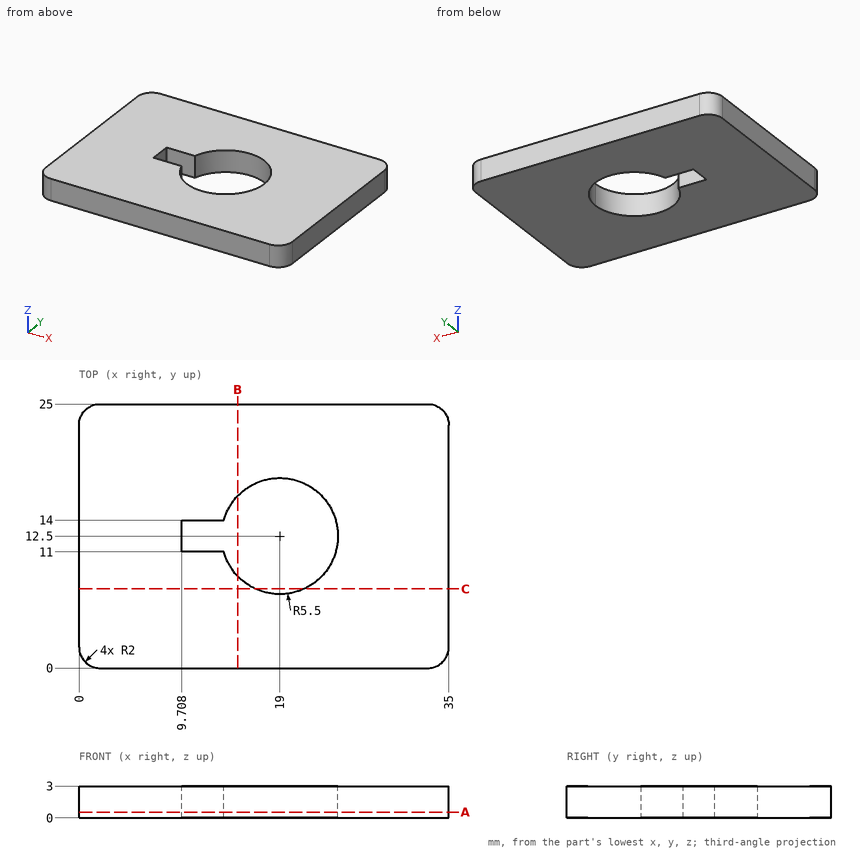
Could you check a few things on this drawing? It's one solid part, dimensions in mm from its lowest x, y, z. Give positions to 0.01 mm unless a question says otherwise; leave off trailing zeros. Write each loop counter-clockwise with the first axis right and the second up, starting at its lowest first coordinate (ties: lowest second). Pieces come first, ordered by that corner, then holes.
(1) If I drill on L1, parallel to X at y = 12.25, z = 2.3 (1 decimal); L2, parallel to Y at x = 19, z = 2.35; L3, parallel to X at y = 13.25, z = 2.05, over which ranges is the centre line in solid material (lowest first)?
Output values:
L1: x = 0 to 9.7, 24.5 to 35
L2: y = 0 to 7, 18 to 25
L3: x = 0 to 9.71, 24.45 to 35
(2) Imagine slicing it at C-C, the plane y = 7.5. Write out the boundary of the cut face in (x, z).
Output values:
outline: (0, 0) - (16.71, 0) - (16.71, 3) - (0, 3) - close; (21.29, 0) - (35, 0) - (35, 3) - (21.29, 3) - close
(3) Imagine slicing it at B-B, the plane x = 15. Write out the boundary of the cut face in (y, z) (1 decimal).
Output values:
outline: (0, 0) - (8.7, 0) - (8.7, 3) - (0, 3) - close; (16.3, 0) - (25, 0) - (25, 3) - (16.3, 3) - close
(4) Imagine slicing it at A-A, the plane z = 0.55. Write out the boundary of the cut face in (x, y).
Output values:
outline: (0, 2) arc R2 ccw to (2, 0) - (33, 0) arc R2 ccw to (35, 2) - (35, 23) arc R2 ccw to (33, 25) - (2, 25) arc R2 ccw to (0, 23) - close; hole (9.71, 11) - (13.71, 11) arc R5.5 ccw (long way) to (13.71, 14) - (9.71, 14) - close
